from build123d import *

# Parameters (mm, degrees)
SKETCH_1_R               = 50
EXTRUDE_1_DEPTH          = 50
CUT_EXTRUDE_2_DEPTH      = 87.602540378
CUT_EXTRUDE_3_DEPTH      = 76
FILLET_1_R               = 2
CHAMFER_1_SIZE           = 0.6
SHELL_1_T                = -1.2
EXTRUDE_2_DEPTH          = 2
EXTRUDE_2_DEPTH_BACK     = 2
SKETCH_4_R               = 1.5
SKETCH_5_R               = 1.5
EXTRUDE_3_DEPTH          = 3
CUT_EXTRUDE_4_DEPTH      = 75.752405905
CUT_EXTRUDE_4_DEPTH_BACK = 75.752405905
SKETCH_7_W               = 6.6
SKETCH_7_H               = 5.6
SKETCH_7_W_2             = 4
SKETCH_7_H_2             = 3
EXTRUDE_4_DEPTH          = 2.2
SKETCH_8_W               = 4
SKETCH_8_H               = 3
CUT_EXTRUDE_7_DEPTH      = 1.2
SKETCH_9_W               = 48.891646461
SKETCH_9_H               = 14.735047163
CUT_EXTRUDE_8_DEPTH      = 75.752405905
CHAMFER_2_SIZE           = 0.4
SKETCH_10_W              = 4.2
SKETCH_10_H              = 3.2
SKETCH_10_W_2            = 4
SKETCH_10_H_2            = 3
CUT_EXTRUDE_9_DEPTH      = 73.52228753
SKETCH_11_W              = 6.6
SKETCH_11_H              = 5.6
EXTRUDE_5_DEPTH          = 1.2


with BuildPart() as part:
    # 草图1 → 凸台-拉伸1 (new body)
    with BuildSketch(Plane(origin=(0, 0, 0), x_dir=(1, 0, 0), z_dir=(0, 1, 0))):
        with Locations(Location((0, 0, 0), (0, 0, 270))):
            Circle(SKETCH_1_R)
    extrude(amount=EXTRUDE_1_DEPTH)

    # 草图2 → 切除-拉伸2 (cut, through all)
    with BuildSketch(Plane(origin=(0, 50, 0), x_dir=(1, 0, 0), z_dir=(0, 1, 0))):
        with BuildLine():
            Line((-25, -43.301270189), (0, 0))
            Line((0, 0), (25, -43.301270189))
            ThreePointArc((25, -43.301270189), (0, 50), (-25, -43.301270189))
        make_face()
    extrude(amount=-CUT_EXTRUDE_2_DEPTH, mode=Mode.SUBTRACT)

    # 草图3 → 切除-拉伸3 (cut, through all)
    with BuildSketch(Plane(origin=(0, 50, 0), x_dir=(1, 0, 0), z_dir=(0, 1, 0))):
        with BuildLine():
            ThreePointArc((-7.5, -12.990381057), (-3.882285677, -14.488887394), (0, -15))
            ThreePointArc((0, -15), (3.882285677, -14.488887394), (7.5, -12.990381057))
            Line((7.5, -12.990381057), (0, 0))
            Line((0, 0), (-7.5, -12.990381057))
        make_face()
        with BuildLine():
            ThreePointArc((15, 0), (-7.5, 12.990381057), (-7.5, -12.990381057))
            Line((-7.5, -12.990381057), (0, 0))
            Line((0, 0), (7.5, -12.990381057))
            ThreePointArc((7.5, -12.990381057), (12.990381057, -7.5), (15, 0))
        make_face()
        with BuildLine():
            ThreePointArc((7.5, -12.990381057), (3.882285677, -14.488887394), (0, -15))
            Line((0, -15), (8.660254038, -15))
            Line((8.660254038, -15), (7.5, -12.990381057))
        make_face()
        with BuildLine():
            Line((-7.5, -12.990381057), (-8.660254038, -15))
            Line((-8.660254038, -15), (0, -15))
            ThreePointArc((0, -15), (-3.882285677, -14.488887394), (-7.5, -12.990381057))
        make_face()
    extrude(amount=-CUT_EXTRUDE_3_DEPTH, mode=Mode.SUBTRACT)

    # 圆角1
    fillet_1_edges = [part.edges().sort_by_distance(p)[0] for p in [
        (25, 25, 43.301270189),
        (-25, 25, 43.301270189),
        (-8.660254038, 25, 15),
        (8.660254038, 25, 15),
    ]]
    fillet(fillet_1_edges, radius=FILLET_1_R)

    # 倒角1
    chamfer_1_edges = [part.edges().sort_by_distance(p)[0] for p in [
        (0, 0, 15),
        (-16.608380962, 0, 28.766559657),
        (16.608380962, 0, 28.766559657),
        (0, 0, 50),
        (8.505553499, 0, 15.267949192),
        (24.167752526, 0, 43.090900659),
        (-24.167752526, 0, 43.090900659),
        (-8.505553499, 0, 15.267949192),
    ]]
    chamfer(chamfer_1_edges, length=CHAMFER_1_SIZE)

    # 抽壳1
    shell_1_openings = [part.faces().sort_by_distance(p)[0] for p in [
        (0, 50, 34.229276229),
    ]]
    offset(amount=SHELL_1_T, openings=shell_1_openings)

    # 草图4 → 凸台-拉伸2 (add, two sides: drawn at the far end of the back side and taken through both)
    with BuildSketch(Plane(origin=(0, 0, 0), x_dir=(0, 0, -1), z_dir=(1, 0, 0)).offset(-EXTRUDE_2_DEPTH_BACK)):
        with BuildLine():
            Line((-44.5, 0), (-44.5, -3))
            ThreePointArc((-44.5, -3), (-43, -1.5), (-41.5, -3))
            Line((-41.5, -3), (-41.5, 0))
            Line((-41.5, 0), (-44.5, 0))
        make_face()
        with Locations((-43, -3)):
            Circle(SKETCH_4_R)
    extrude(amount=EXTRUDE_2_DEPTH + EXTRUDE_2_DEPTH_BACK)

    # 草图5 → 凸台-拉伸3 (add)
    with BuildSketch(Plane(origin=(2, 0, 0), x_dir=(0, 0, -1), z_dir=(1, 0, 0))):
        with Locations((-43, -3)):
            Circle(SKETCH_5_R)
    extrude_3 = extrude(amount=EXTRUDE_3_DEPTH)

    # 镜向1: 凸台-拉伸3 across plane
    add(extrude_3.mirror(Plane(origin=(0, 0, 0), x_dir=(0, 0, 1), z_dir=(1, 0, 0))))

    # 草图6 → 切除-拉伸4 (cut, two sides: drawn at the far end of the back side and taken through both)
    with BuildSketch(Plane(origin=(0, 0, 0), x_dir=(0, 0, -1), z_dir=(1, 0, 0)).offset(-CUT_EXTRUDE_4_DEPTH_BACK)):
        with BuildLine():
            ThreePointArc((-41.533119315, 49.979696687), (-27.735886723, 47.754377603), (-15, 42))
            Line((-15, 42), (-15, 50))
            Line((-15, 50), (-16, 50))
            Line((-16, 50), (-41.533119315, 50))
            Line((-41.533119315, 50), (-41.533119315, 49.979696687))
        make_face()
    extrude(amount=CUT_EXTRUDE_4_DEPTH + CUT_EXTRUDE_4_DEPTH_BACK, mode=Mode.SUBTRACT)

    # 草图7 → 凸台-拉伸4 (add)
    with BuildSketch(Plane(origin=(0, 1.2, 0), x_dir=(1, 0, 0), z_dir=(0, 1, 0))):
        with Locations((0, -43)):
            Rectangle(SKETCH_7_W, SKETCH_7_H)
        with Locations((0, -43)):
            Rectangle(SKETCH_7_W_2, SKETCH_7_H_2, mode=Mode.SUBTRACT)
    extrude(amount=EXTRUDE_4_DEPTH)

    # 草图8 → 切除-拉伸7 (cut)
    with BuildSketch(Plane(origin=(0, 1.2, 0), x_dir=(1, 0, 0), z_dir=(0, 1, 0))):
        with Locations((0, -43)):
            Rectangle(SKETCH_8_W, SKETCH_8_H)
    extrude(amount=-CUT_EXTRUDE_7_DEPTH, mode=Mode.SUBTRACT)


with BuildPart() as cut_extrude_7_piece_1:
    # of the separate pieces the step leaves, piece 1, a body of its own (cut_extrude_7_pieces)
    add(part.part.solids().sort_by_distance((-23.174069593, 0.6, 44.305332619))[0])

    # 倒角2
    chamfer_2_edges = [cut_extrude_7_piece_1.edges().sort_by_distance(p)[0] for p in [
        (-2, 0, 43),
        (0, 0, 41.5),
        (0, 0, 44.5),
        (2, 0, 43),
    ]]
    chamfer(chamfer_2_edges, length=CHAMFER_2_SIZE)

    # 草图10 → 切除-拉伸9 (cut, through all)
    with BuildSketch(Plane(origin=(0, 3.4, 0), x_dir=(1, 0, 0), z_dir=(0, 1, 0))):
        with Locations((0, -43)):
            Rectangle(SKETCH_10_W, SKETCH_10_H)
        with Locations((0, -43)):
            Rectangle(SKETCH_10_W_2, SKETCH_10_H_2, mode=Mode.SUBTRACT)
    extrude(amount=-CUT_EXTRUDE_9_DEPTH, mode=Mode.SUBTRACT)

    # 草图11 → 凸台-拉伸5 (add)
    with BuildSketch(Plane(origin=(0, 3.4, 0), x_dir=(1, 0, 0), z_dir=(0, 1, 0))):
        with Locations((0, -43)):
            Rectangle(SKETCH_11_W, SKETCH_11_H)
    extrude(amount=EXTRUDE_5_DEPTH)


with BuildPart() as cut_extrude_7_piece_2:
    # of the separate pieces the step leaves, piece 2, a body of its own (cut_extrude_7_pieces)
    add(part.part.solids().sort_by_distance((-2, -3, 41.5))[0])

    # 草图9 → 切除-拉伸8 (cut, through all)
    with BuildSketch(Plane.XZ):
        with Locations((-1.815492917, 42.673305219)):
            Rectangle(SKETCH_9_W, SKETCH_9_H)
    extrude(amount=CUT_EXTRUDE_8_DEPTH, mode=Mode.SUBTRACT)


solid = cut_extrude_7_piece_1.part
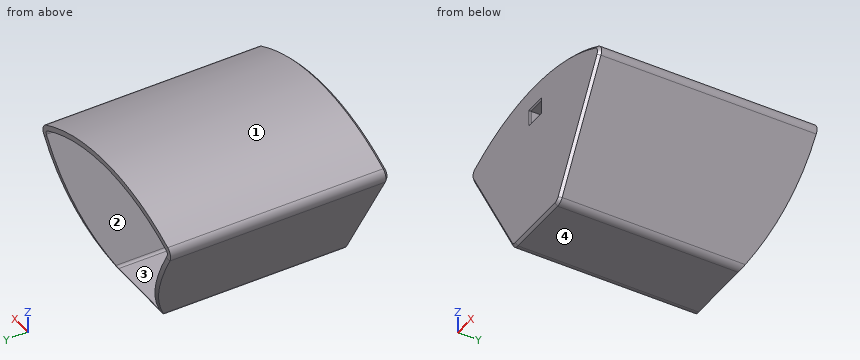
Input: part model. Units: mm. Frame: model coordinates. Face numbers are marked on the shaded views. Give positions to 0.01 mm unless a question says otherwise; leave off trailing zeros. Loops run counter-clockwise (first coordinate to the right, second up) from the corner with the lowest first, then second, coordinate; pieces in that order, holes last. Notation, with made-up numbers: (78, 11) - (102, 11) arc R19 cw to (102, 31) - close; hole circle Ø1 at (24, -37). An arc over 180 degrees is marked (long way). Use CSV: the item, a comma, the result in double quotes. Start each with the question number.
Item 1: Section A-A on y = 6.5. Return loops of the section in (x, z), then the cut area to 3 significant figures.
Item 2: Contact query for flat-ended pins moving along their axis: P1, Ø2, axis at x = 16, z = 26, coming from the +Y side; P2, Ø10, axis at x = 5.5, y = 9, coming from the +Z side; P3, Ø1, axis at x = 19.5, y = 17.5, coming from the +Z side. Output: stop coordinate, or through.
Item 3: Mould query, pull axis X, two halves, no side actions, for the marked faces 1, 2, 3 and 4. Classes: pulls with the +X half, pulls with the -X half, needs draft (parallel to the pull), parting line crosses it, or undercut.
Item 4: Section C-C on y = 44. Return loops of the section in (x, z), then the cut area to 3 significant figures.
Item 5: Section D-D on z = 18. Return loops of the section in (x, y), then the cut area to 3 significant figures.
Item 6: Section B-B on z = 27. Return loops of the section in (x, y), then the cut area to 3 significant figures.
Item 7: Line query: line 1 (Z direction, x = -2.5, y = 2); line 2 (Y direction, x = -1, z = 26); line 3 (Z direction, x = -9.5, y = 19.5). Output: solid intervals per line, ascending.
Ans:
1,outline,"(-23.98, 41.53) - (-9.24, 16) arc R2 ccw to (-7.51, 15) - (7.51, 15) arc R2 ccw to (9.24, 16) - (23.98, 41.53) arc R2 ccw to (23.17, 44.31) arc R50 ccw to (-23.17, 44.31) arc R2 ccw to start; hole (-22.94, 42.13) - (-8.2, 16.6) arc R0.8 ccw to (-7.51, 16.2) - (7.51, 16.2) arc R0.8 ccw to (8.2, 16.6) - (22.94, 42.13) arc R0.8 ccw to (22.62, 43.24) arc R48.8 ccw to (-22.62, 43.24) arc R0.8 ccw to start"
1,area,"155 mm2"
2,P1,"stops at y = 47.49"
2,P2,"stops at z = 50"
2,P3,"stops at z = 46.25"
3,face 1,"parting line crosses it"
3,face 2,"undercut"
3,face 3,"undercut"
3,face 4,"needs draft"
4,outline,"(-23.98, 41.53) - (-10.68, 18.51) - (-9.3, 18.51) - (-22.94, 42.13) arc R0.8 cw to (-22.62, 43.24) arc R48.8 cw to (22.62, 43.24) arc R0.8 cw to (22.94, 42.13) - (9.3, 18.51) - (10.68, 18.51) - (23.98, 41.53) arc R2 ccw to (23.17, 44.31) arc R50 ccw to (-23.17, 44.31) arc R2 ccw to start"
4,area,"127 mm2"
5,outline,"(-10.39, 0.6) - (-9.7, 0) - (9.7, 0) - (10.39, 0.6) - (10.39, 43.73) - (9.01, 43.73) - (9.01, 1.2) - (-9.01, 1.2) - (-9.01, 43.73) - (-10.39, 43.73) - close"
5,area,"142 mm2"
6,outline,"(-15.59, 0.6) - (-14.9, 0) - (14.9, 0) - (15.59, 0.6) - (15.59, 47.53) - (14.2, 47.53) - (14.2, 1.2) - (-14.2, 1.2) - (-14.2, 47.53) - (-15.59, 47.53) - close"
6,area,"165 mm2"
7,line 1,"z = 15 to 16.2, 40.2 to 45.8, 48.74 to 49.94"
7,line 2,"y = 0 to 1.2"
7,line 3,"z = 16.45 to 18.85, 47.87 to 49.09"
